Autodesk Inventor part; units mm, degrees
ref_plane "YZ Plane" through (0, 0, 0) normal (1, 0, 0) x (0, 1, 0)
ref_plane "XZ Plane" through (0, 0, 0) normal (0, 1, 0) x (-1, 0, 0)
ref_plane "XY Plane" through (0, 0, 0) normal (0, 0, 1) x (1, 0, 0)
sketch "Эскиз1" plane through (0, 0, 0) normal (0, 0, 1) x (1, 0, 0)
  line L0 (0, 0) -> (0, 26)
  line L1 (9, 26.1456) -> (9, 30.5)
  line L2 (9, 30.5) -> (14.45, 30.5)
  line L3 (14.45, 30.5) -> (14.45, 17.5)
  line L4 (14.45, 17.5) -> (10, 17.5)
  line L5 (10, 17.5) -> (10, 0)
  line L6 (10, 0) -> (0, 0)
  line L7 (0, 26) -> (3.5, 26)
  line L8 (3.5, 26) -> (4, 25.5)
  line L9 (4, 25.5) -> (9, 25.5)
  line L10 (9, 25.5) -> (9, 26.1456)
  dimension "d1" = 52
  dimension "d2" = 0.5
  dimension "d3" = 45
  dimension "d4" = 5
  dimension "d5" = 14.45
  dimension "d6" = 10
  dimension "d7" = 35
  dimension "d8" = 4.5
  dimension "d23" = 9
revolve "Вращение1" add sketch "Эскиз1" angle 360 about axis through (10, 0, 0) along (-1, 0, 0)
sketch "Эскиз2" plane through (0, 0, 0) normal (-1, 0, 0) x (0, 0, 1)
  circle A0 centre (0, 0) radius 26
  circle A1 centre (0, 0) radius 10
  circle A2 centre (0, 0) radius 5
  point P0 (0, 0)
  dimension "d10" = 20
  dimension "d11" = 10
extrude "Выдавливание1" cut sketch "Эскиз2" against normal through all contours A2
fillet "Сопряжение2" radius 0.5 1 edges at (4, -25.5, 0)
chamfer "Фаска2" distance 1 angle 45 1 edges at (0, 0, -5)
thread "Резьба3"
properties part number "Крышка_пром_новая"
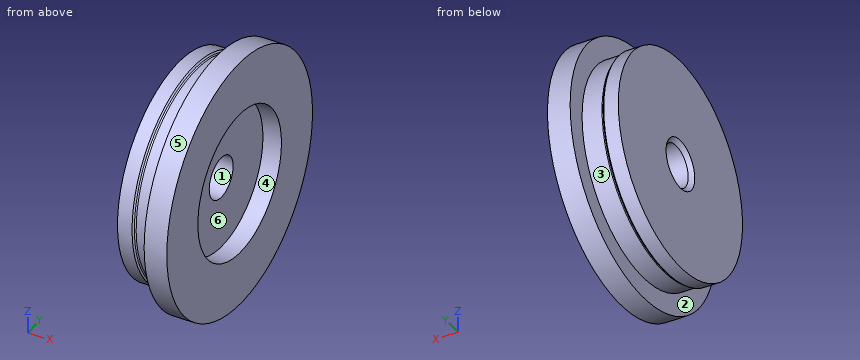
Part model, mm, in its own coordinate system. Face numbers are marked on the shaded views. A direction names the side the tool comes from. Round coordinates to 2 decimals unless told otherwise and drop trailing zeros. Use one line per item in the form item = value. Start each with the question number.
Item 1: Drill centre lines: line 1 along Y through (x, z) = (5.5, 0); line 2 along Z through (x, y) = (11.5, 0); line 3 along X through (y, z) = (11, 5). Where is each one in solid material? Low to high.
Item 2: Tool access for the marked faces 5 and 6: list every direction of +Z, -Z, +X, -X, +Y, -Y with a clear straight run to the whole face (end or side of a thin tool).
Item 3: Drop flat-ended pins along their axis: pin 1 Ø6 at (x, y) = (4, 3.5) entering from -Z; pin 2 Ø4 at (x, z) = (6.5, 7.5) entering from +Y; pin 3 Ø6 at (y, z) = (0, 0) entering from +X (3 decimals); pin 4 Ø4 at (x, y) = (13, 6.5) entering from -Z. Give the stop position or say it passes through.
Item 4: Two-plate mould, pull along Z, no slides. Class the marked faces 1, 2, 3 and 4: released by +Z, released by -Z, zero draft, split by the parting line, or undercut.
Data:
q1.line_1 = -25.5 to -5, 5 to 25.5
q1.line_2 = -30.5 to -17.5, 17.5 to 30.5
q1.line_3 = 0 to 10
q2.face_5 = +X, -X
q2.face_6 = +X
q3.pin_1 = -25.99
q3.pin_2 = 24.9
q3.pin_3 = through
q3.pin_4 = -30.17
q4.face_1 = undercut
q4.face_2 = zero draft
q4.face_3 = split by the parting line
q4.face_4 = undercut
